CAD build for the part. Positions are in the model's coordinates, mm. Coordinates: 2 decimals unless noted, no trailing zeros. Order: outer loops, then holes, each group sorted by start corner. A loop starts at its lowest first (then second) coordinate and runs counter-clockwise, first axis right, second up.
from build123d import *

# Parameters (mm, degrees)
F1_DEPTH = 1.5
F3_W     = 24
F3_H     = 1.5
F4_DEPTH = 14
F5_R     = 1.49999


# Not quite as in the source:
# - a fillet or chamfer is up to 0.001 mm smaller than in the source, because OpenCascade refuses the exact size


with BuildPart() as f1:
    # F0 (on Top) → F1 (new body)
    with BuildSketch(Plane.XY):
        with BuildLine():
            Line((375, 14), (25, 14))
            Line((25, 14), (25, 0))
            Line((25, 0), (0, 0))
            Line((0, 0), (0, -26))
            ThreePointArc((0, -26), (15, -41), (0, -56))
            Line((0, -56), (0, -82))
            Line((0, -82), (25, -82))
            Line((25, -82), (25, -96))
            Line((25, -96), (375, -96))
            Line((375, -96), (375, -82))
            Line((375, -82), (400, -82))
            Line((400, -82), (400, -56))
            ThreePointArc((400, -56), (385, -41), (400, -26))
            Line((400, -26), (400, 0))
            Line((400, 0), (375, 0))
            Line((375, 0), (375, 14))
        make_face()
    extrude(amount=F1_DEPTH)

    # F3 (on face) → F4 (join)
    with BuildSketch(Plane.XY.offset(1.5)):
        with Locations((12, -0.75)):
            Rectangle(F3_W, F3_H)
        with Locations((388, -0.75)):
            Rectangle(F3_W, F3_H)
        with Locations((12, -81.25)):
            Rectangle(F3_W, F3_H)
        with Locations((388, -81.25)):
            Rectangle(F3_W, F3_H)
    extrude(amount=F4_DEPTH)

    # F5 (radius 1.5 in the source; OpenCascade refuses exactly that, so slightly less here)
    f5_edges = [f1.edges().sort_by_distance(p)[0] for p in [
        (12.5, 0, 0),
        (12.5, -82, 0),
        (387.5, -82, 0),
        (387.5, 0, 0),
    ]]
    fillet(f5_edges, radius=F5_R)


solid = f1.part
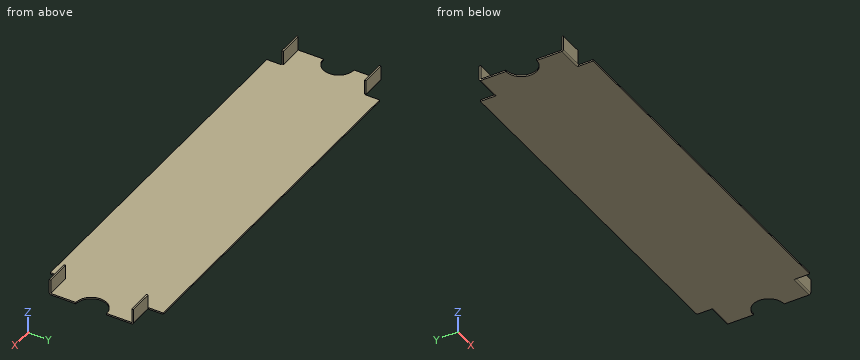
1) Pin check, flat tips, straight feed: P1, Ø3, axis at x = 312, y = -31, coming from the +Z side; P2, Ø0.5, axis at y = 5, z = 0.5, coming from the +X side; P3, Ø7, axis at x = 387.5, z = 7, coming from the +Y side. Stop position of each tip, or through.
2) Drill centre lines: probe 1 along Z at (x, y) = (54.5, -64); probe 2 along X at (y, z) = (-49, 1); probe 3 along X at (y, z) = (-44, 1.25). Where is each one in solid material? Low to high.
3) Slice it at A-A (z = 9). List the corners of the cut face in (x, y).
4) Slice it at C-C (y = -41). List the corners of the cut face in (x, z).
5) Slice it at B-B (x = 92). List the corners of the cut face in (y, z), plus the area to 3 significant figures.
Worked out:
1. P1: stops at z = 1.5
1. P2: stops at x = 375
1. P3: stops at y = 0
2. probe 1: z = 0 to 1.5
2. probe 2: x = 12.69 to 387.31
2. probe 3: x = 14.7 to 385.3
3. outline: (0, -82) - (24, -82) - (24, -80.5) - (0, -80.5) - close; (0, -1.5) - (24, -1.5) - (24, 0) - (0, 0) - close; (376, -82) - (400, -82) - (400, -80.5) - (376, -80.5) - close; (376, -1.5) - (400, -1.5) - (400, 0) - (376, 0) - close
4. outline: (15, 0) - (385, 0) - (385, 1.5) - (15, 1.5) - close
5. outline: (-96, 0) - (14, 0) - (14, 1.5) - (-96, 1.5) - close
5. area: 165 mm2
